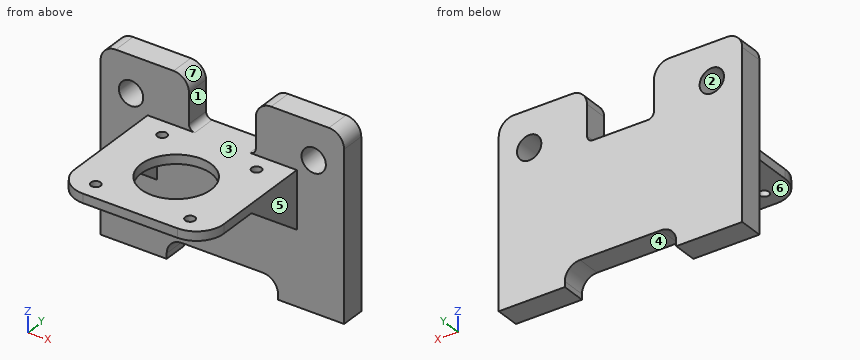
```python
from build123d import *

# Parameters (mm, degrees)
F0_R     = 5
F0_R_2   = 4
F1_DEPTH = 8
F2_W     = 49
F2_H     = 43
F2_R     = 1.6
F2_R_2   = 11.5
F3_DEPTH = 3
F5_DEPTH = 3
F6_R     = 9
F8_DEPTH = 3
F9_DEPTH = 8


# Not quite as in the source:
# - a feature of the source that left no trace in its solid (it failed there, or was rolled back) is left out


with BuildPart() as f1:
    # F0 (on Front) → F1 (new body)
    with BuildSketch(Plane.XZ):
        with BuildLine():
            Line((-15.9509392173, 58.3590910856), (-34.9509392173, 58.3590910856))
            ThreePointArc((-34.9509392173, 58.3590910856), (-38.4864731233, 56.8946249915), (-39.9509392173, 53.3590910856))
            Line((-39.9509392173, 53.3590910856), (-39.9509392173, -1.6409089144))
            Line((-39.9509392173, -1.6409089144), (-18.2393845171, -1.6409089144))
            Line((-18.2393845171, -1.6409089144), (-18.2393845171, 0.1278397727))
            ThreePointArc((-18.2393845171, 0.1278397727), (-16.774918423, 3.6633736787), (-13.2393845171, 5.1278397727))
            Line((-13.2393845171, 5.1278397727), (13.3375060824, 5.1278397727))
            ThreePointArc((13.3375060824, 5.1278397727), (16.8730399883, 3.6633736787), (18.3375060824, 0.1278397727))
            Line((18.3375060824, 0.1278397727), (18.3375060824, -1.6409089144))
            Line((18.3375060824, -1.6409089144), (40.0490607827, -1.6409089144))
            Line((40.0490607827, -1.6409089144), (40.0490607827, 53.3590910856))
            ThreePointArc((40.0490607827, 53.3590910856), (38.5845946886, 56.8946249915), (35.0490607827, 58.3590910856))
            Line((35.0490607827, 58.3590910856), (16.0490607827, 58.3590910856))
            ThreePointArc((16.0490607827, 58.3590910856), (12.5135268767, 56.8946249915), (11.0490607827, 53.3590910856))
            Line((11.0490607827, 53.3590910856), (11.0490607827, 43.3590910856))
            ThreePointArc((11.0490607827, 43.3590910856), (10.463274345, 41.9448775232), (9.0490607827, 41.3590910856))
            Line((9.0490607827, 41.3590910856), (-8.9509392173, 41.3590910856))
            ThreePointArc((-8.9509392173, 41.3590910856), (-10.3651527797, 41.9448775232), (-10.9509392173, 43.3590910856))
            Line((-10.9509392173, 43.3590910856), (-10.9509392173, 53.3590910856))
            ThreePointArc((-10.9509392173, 53.3590910856), (-12.4154053114, 56.8946249915), (-15.9509392173, 58.3590910856))
        make_face()
        with Locations((-29.9509392173, 10.3590910856)):
            Circle(F0_R, mode=Mode.SUBTRACT)
        with Locations((30.0490607827, 10.3590910856)):
            Circle(F0_R, mode=Mode.SUBTRACT)
        with Locations((-29.9509392173, 46.3590910856)):
            Circle(F0_R_2, mode=Mode.SUBTRACT)
        with Locations((30.0490607827, 46.3590910856)):
            Circle(F0_R_2, mode=Mode.SUBTRACT)
    extrude(amount=F1_DEPTH)

    # F2 (on face) → F3 (join)
    with BuildSketch(Plane.XY.offset(41.3590910856)):
        with Locations((0.0111820996, -29.5)):
            Rectangle(F2_W, F2_H)
        with Locations((-15.5, -45)):
            Circle(F2_R, mode=Mode.SUBTRACT)
        with Locations((15.5, -45)):
            Circle(F2_R, mode=Mode.SUBTRACT)
        with Locations((0, -29.5)):
            Circle(F2_R_2, mode=Mode.SUBTRACT)
        with Locations((-15.5, -14)):
            Circle(F2_R, mode=Mode.SUBTRACT)
        with Locations((15.5, -14)):
            Circle(F2_R, mode=Mode.SUBTRACT)
    extrude(amount=-F3_DEPTH)

    # F4 (on face) → F5 (join)
    with BuildSketch(Plane(origin=(-24.4888179004, 0, 0), x_dir=(0, -1, 0), z_dir=(-1, 0, 0))):
        Polygon((29.5, 38.3590910856), (8, 38.3590910856), (7.8833866864, 22.056709975), align=None)
    extrude(amount=-F5_DEPTH)

    # F6
    f6_edges = [f1.edges().sort_by_distance(p)[0] for p in [
        (-24.488818, -51, 39.859091),
        (24.511182, -51, 39.859091),
    ]]
    fillet(f6_edges, radius=F6_R)

    # F7 (on face) → F8 (join)
    with BuildSketch(Plane.YZ.offset(24.5111820996)):
        Polygon((-8, 38.3590910856), (-29.1853044182, 38.3590910856), (-8, 22.5599054247), align=None)
    extrude(amount=-F8_DEPTH)

    # F0 (on Front) → F9 (join)
    with BuildSketch(Plane.XZ):
        with Locations((30.0490607827, 10.3590910856)):
            Circle(F0_R)
        with Locations((-29.9509392173, 10.3590910856)):
            Circle(F0_R)
    extrude(amount=F9_DEPTH)


with BuildPart() as f10_1:
    # F10: copy of F1
    add(f1.part)


solid = f1.part
```
CAD build for the part. Positions are in the model's coordinates, mm. Face numbers are marked on the shaded views. A direction names the side the tool comes from. Round coordinates to 2 decimals unless told otherwise and drop trailing zeros. Order: outer loops, then holes, each group sorted by start corner. A loop starts at its lowest first (then second) coordinate and runs counter-clockwise, first axis right, second up. Notation, with made-up numbers: (15.25, 69.25) -> (68.25, 69.25) arc R23 cw to (68.25, 96.25) -> close; hole circle Ø2 at (9.25, -33). An arc over 180 degrees is marked (long way). One line per question, with ' | ' between items.
Q1. Two-plate mould, pull along Z, no slides. Class the marked faces 1, 2 and 3: released by +Z, released by -Z, zero draft, split by the parting line, or undercut.
Completed:
face 1: zero draft | face 2: undercut | face 3: released by +Z
Q2. Slice it at A-A (x = 0). Write the cut outline in (y, z), then the cut area to 3 significant figures.
Completed:
outline: (-51, 38.36) -> (-41, 38.36) -> (-41, 41.36) -> (-51, 41.36) -> close; (-18, 38.36) -> (-8, 38.36) -> (-8, 5.13) -> (0, 5.13) -> (0, 41.36) -> (-18, 41.36) -> close | area: 350 mm^2
Q3. Probe probe 1 along Y at (x, z) = (15.5, 40); probe 2 along Y at (x, z) = (0, 39); probe 3 along Y at (x, z) = (15, 39). List the from-to ranges inside material, lowest first.
Completed:
probe 1: y = -51 to -46.6, -43.4 to -15.6, -12.4 to 0 | probe 2: y = -51 to -41, -18 to 0 | probe 3: y = -51 to -46.52, -43.48 to -15.52, -12.48 to 0
Q4. Slice it at C-C (z = 48). Write the cut outline in (x, y), then the cut area to 3 significant figures.
Completed:
outline: (-39.95, -8) -> (-33.6, -8) -> (-33.6, 0) -> (-39.95, 0) -> close; (-26.3, -8) -> (-10.95, -8) -> (-10.95, 0) -> (-26.3, 0) -> close; (11.05, -8) -> (26.4, -8) -> (26.4, 0) -> (11.05, 0) -> close; (33.7, -8) -> (40.05, -8) -> (40.05, 0) -> (33.7, 0) -> close | area: 347 mm^2
Q5. Slice it at B-B (y = -14). Write the cut outline in (x, z).
Completed:
outline: (-24.49, 26.67) -> (-21.49, 26.67) -> (-21.49, 38.36) -> (-17.1, 38.36) -> (-17.1, 41.36) -> (-24.49, 41.36) -> close; (-13.9, 38.36) -> (13.9, 38.36) -> (13.9, 41.36) -> (-13.9, 41.36) -> close; (17.1, 38.36) -> (21.51, 38.36) -> (21.51, 27.03) -> (24.51, 27.03) -> (24.51, 41.36) -> (17.1, 41.36) -> close
Q6. Which spindle directions (+Z, -Z, +X, -X, +Y, -Y) get a long thin tool onto all of the face, cutting with end or side? Do the marked faces 4, 5, 6 and 7. Say none if no direction does.
Completed:
face 4: -Z, +Y, -Y | face 5: +Z, -Z, +X, -Y | face 6: -Z, -Y | face 7: +Z, +Y, -Y
Q7. Drop flat-ended pins along their axis: pin 1 (5 mm diameter, centred on x = -15.5, y = -45, fed in from -Z); pin 2 (3.5 mm diameter, centred on x = 15.5, y = -45, fed in from +Z); pin 3 (2.5 mm diameter, centred on x = -6, y = -4.5, fed in from -Z); pin 4 (1.9 mm diameter, centred on x = -15.5, y = -14, fed in from +Z). Give the stop position or say it passes through.
Completed:
pin 1: stops at z = 38.36 | pin 2: stops at z = 41.36 | pin 3: stops at z = 5.13 | pin 4: passes through
Q8. Slice it at D-D (y = -23.5). Write the cut outline in (x, z), then the cut area to 3 significant figures.
Completed:
outline: (-24.49, 33.83) -> (-21.49, 33.83) -> (-21.49, 38.36) -> (-9.81, 38.36) -> (-9.81, 41.36) -> (-24.49, 41.36) -> close; (9.81, 38.36) -> (21.51, 38.36) -> (21.51, 34.12) -> (24.51, 34.12) -> (24.51, 41.36) -> (9.81, 41.36) -> close | area: 114 mm^2
